```python
from build123d import *

# Parameters (mm, degrees)
F1_DEPTH = 20
F2_R     = 5
F3_R     = 0.99999
F4_R     = 3


# Not quite as in the source:
# - a fillet or chamfer is up to 0.001 mm smaller than in the source, because OpenCascade refuses the exact size


with BuildPart() as f1:
    # F0 (on Top) → F1 (new body)
    with BuildSketch(Plane.XY):
        Polygon((0, 18), (0, 0), (2, 0), (2, 16), (22.5, 16), (22.5, -17), (41.5, -17), (41.5, 0), (39.5, 0), (39.5, -12), (24.5, -12), (24.5, 18), align=None)
    extrude(amount=F1_DEPTH)

    # F2
    f2_edges = [f1.edges().sort_by_distance(p)[0] for p in [
        (40.5, 0, 20),
        (40.5, 0, 0),
    ]]
    fillet(f2_edges, radius=F2_R)

    # F3 (radius 1 in the source; OpenCascade refuses exactly that, so slightly less here)
    f3_edges = [f1.edges().sort_by_distance(p)[0] for p in [
        (0, 18, 10),
        (24.5, 18, 10),
        (2, 0, 10),
        (22.5, -17, 10),
        (41.5, -17, 10),
        (0, 0, 10),
    ]]
    fillet(f3_edges, radius=F3_R)

    # F4
    f4_edges = [f1.edges().sort_by_distance(p)[0] for p in [
        (24.5, -12, 10),
        (39.5, -12, 10),
    ]]
    fillet(f4_edges, radius=F4_R)


solid = f1.part
```
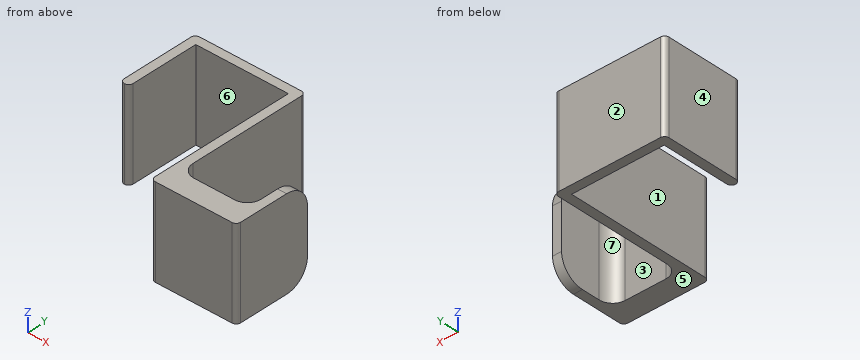
For this review, take the finished solid that the model builds, in its own axes (mm). Face numbers are marked on the shaded views. A direction names the side the tool comes from. Round coordinates to 2 decimals unless told otherwise and drop trailing zeros. Order: outer loops, then holes, each group sorted by start corner. A loop starts at its lowest first (then second) coordinate and runs counter-clockwise, first axis right, second up. Notation, with made-up numbers: (10, 78.5) -> (27, 78.5) arc R20 cw to (27, 90.5) -> close; hole circle Ø5 at (4.25, -30). An arc over 180 degrees is marked (long way). Use a Markdown table: item, result.
Item 1: For pin 1 (6 mm diameter, centred on x = 18.5, z = 6.5, fed in from -Y); pin 2 (4.5 mm diameter, centred on y = -3.5, z = 10, fed in from -X); pin 3 (2 mm diameter, centred on x = 40, z = 9.5, fed in from +Y), all flat-tipped, find the tip position at first contact; note any pin that passes through.
Resolved:
| item | result |
|---|---|
| pin 1 | stops at y = 16 |
| pin 2 | stops at x = 22.5 |
| pin 3 | stops at y = 0 |
Item 2: Take a section at D-D (y = 9.5). State the section outline as (x, z) points.
Resolved:
| item | result |
|---|---|
| outline | (0, 0) -> (2, 0) -> (2, 20) -> (0, 20) -> close; (22.5, 0) -> (24.5, 0) -> (24.5, 20) -> (22.5, 20) -> close |
Item 3: For line 1 along X through (y, z) = (15, 8.75); line 2 along X through (y, z) = (-8, 12.75); line 3 along Y through (x, z) = (15.5, 16.5), list the stretches that pass through material, from the lowest coordinate up. Write a range as [from, to].
Resolved:
| item | result |
|---|---|
| line 1 | x = [0, 2], [22.5, 24.5] |
| line 2 | x = [22.5, 24.5], [39.5, 41.5] |
| line 3 | y = [16, 18] |
Item 4: Machinability: for the marked faces 1, 2 and 3, which of the approach directions +Z, -Z, +X, -X, +Y, -Y give a long, thin tool a straight path to every point of the face, cutting with its end or side? Answer none if there is none.
Resolved:
| item | result |
|---|---|
| face 1 | +Z, -Z, -Y |
| face 2 | +Z, -Z, +X, -X, +Y |
| face 3 | +Z, -Z, +Y |
Item 5: Take a section at A-A (y = -2). State the section outline as (x, z) points.
Resolved:
| item | result |
|---|---|
| outline | (22.5, 0) -> (24.5, 0) -> (24.5, 20) -> (22.5, 20) -> close; (39.5, 1) -> (41.5, 1) -> (41.5, 19) -> (39.5, 19) -> close |
Item 6: Take a section at C-C (x = 16.5). State the section outline as (y, z) points, plus the area to 3 significant figures.
Resolved:
| item | result |
|---|---|
| outline | (16, 0) -> (18, 0) -> (18, 20) -> (16, 20) -> close |
| area | 40.0 mm² |
Item 7: Draft analysis for pull direction X (two halves, no side actions). For the marked faces 4, 5, 6 and 7, state which applies: +X half, -X half, draft (parallel to the pull), parting line (faces both ways), or undercut.
Resolved:
| item | result |
|---|---|
| face 4 | -X half |
| face 5 | draft |
| face 6 | undercut |
| face 7 | undercut |
